Could you check a few things on this model? Use its own coordinates, in mm. Face numbers are marked on the shaded views. Coordinates: 2 decimals unless noted, no trailing zeros. Loops run counter-clockwise (first coordinate to the right, second up) from the corner with the lowest first, then second, coordinate; pieces in that order, holes last. Notation, with made-up numbers: (51.25, 42) - (68.25, 42) arc R17 ccw to (68.25, 69) - close; hole circle Ø3 at (-7, -19.5). An arc over 180 degrees is marked (long way). Put each result on its own line as item: value. Start each with the question number.
Autodesk Inventor part; units mm, degrees
ref_plane "YZ Plane" through (0, 0, 0) normal (1, 0, 0) x (0, 1, 0)
ref_plane "XZ Plane" through (0, 0, 0) normal (0, 1, 0) x (-1, 0, 0)
ref_plane "XY Plane" through (0, 0, 0) normal (0, 0, 1) x (1, 0, 0)
sketch "Sketch1" plane through (0, 0, 0) normal (0, 1, 0) x (-1, 0, 0)
  line L0 (113.8016, -163.8079) -> (118.6285, -172.1682)
  line L1 (113.8016, -163.8079) -> (118.4883, -163.8079)
  arc A0 (32.1771, -413.0024) -> (33.3318, -411.0024) centre (32.1771, -411.669) ccw
  line L2 (26.4886, -397.8099) -> (26.4886, -373.629)
  arc A1 (26.4886, -370.9624) -> (26.4886, -373.629) centre (26.4886, -372.2957) ccw
  line L3 (26.4886, -370.9624) -> (32.9886, -370.9624)
  arc A2 (32.9886, -373.629) -> (32.9886, -370.9624) centre (32.9886, -372.2957) ccw
  line L4 (32.9886, -373.629) -> (32.9886, -380.9624)
  line L5 (-88.7072, -380.9624) -> (-33.5061, -380.9624)
  line L6 (32.9886, -380.9624) -> (90.3221, -380.9624)
  arc A3 (-33.9776, -411.0024) -> (-32.8229, -413.0024) centre (-32.8229, -411.669) ccw
  arc A4 (-27.1344, -373.6228) -> (-27.0061, -370.9624) centre (-27.0061, -372.2957) ccw
  line L7 (-27.0061, -370.9624) -> (-33.5061, -370.9624)
  arc A5 (-33.5061, -370.9624) -> (-33.5061, -373.629) centre (-33.5061, -372.2957) ccw
  line L8 (-33.5061, -373.629) -> (-33.5061, -380.9624)
  line L9 (118.4883, -148.1364) -> (118.4883, -161.1412)
  line L10 (33.3318, -411.0024) -> (27.1585, -400.3099)
  arc A6 (26.4886, -397.8099) -> (27.1585, -400.3099) centre (31.4886, -397.8099) ccw
  line L11 (-27.1344, -397.8099) -> (-27.1344, -373.6228)
  line L12 (-33.9776, -411.0024) -> (-27.8043, -400.3099)
  arc A7 (-27.8043, -400.3099) -> (-27.1344, -397.8099) centre (-32.1344, -397.8099) ccw
  line L13 (-32.8229, -413.0024) -> (32.1771, -413.0024)
  line L14 (-11.4601, -148.0629) -> (-11.4601, -168.7264)
  line L15 (156.6836, -142.6364) -> (162.6836, -142.6364)
  line L16 (162.6836, -142.6364) -> (162.6836, -148.1364)
  line L17 (156.6866, -148.1364) -> (118.4883, -148.1364)
  line L18 (11.6836, -145.4697) -> (11.6846, -142.6364)
  line L19 (11.6846, -142.6364) -> (5.6846, -142.6364)
  line L20 (5.6846, -142.6364) -> (5.6845, -148.1281)
  line L21 (11.6831, -148.1364) -> (49.8814, -148.1364)
  arc A8 (11.6836, -145.4697) -> (11.6831, -148.1364) centre (11.6831, -146.803) ccw
  arc A9 (3.0194, -148.0629) -> (5.6845, -148.1281) centre (4.3512, -148.1281) ccw
  line L22 (-11.4601, -148.0629) -> (3.0194, -148.0629)
  line L23 (-11.4601, -171.393) -> (-18.9601, -171.393)
  arc A10 (-11.4601, -171.393) -> (-11.4601, -168.7264) centre (-11.4601, -170.0597) ccw
  line L24 (162.6836, -145.3864) -> (185.043, -145.3864) construction
  line L25 (21.6753, -413.0028) -> (-28.7481, -413.0028) construction
  line L26 (-0.3229, -413.0028) -> (-0.3229, -413.0028)
  arc A11 (-89.9069, -379.0472) -> (-88.7072, -380.9624) centre (-88.7072, -379.629) ccw
  line L27 (156.6836, -142.6364) -> (156.6836, -145.4697)
  line L28 (165.3503, -148.1364) -> (179.8299, -148.1364)
  arc A12 (156.6866, -148.1364) -> (156.6836, -145.4697) centre (156.6836, -146.803) ccw
  arc A13 (162.6836, -148.1364) -> (165.3503, -148.1364) centre (164.017, -148.1364) ccw
  line L29 (179.8299, -148.1364) -> (179.8299, -171.4697)
  line L30 (179.8299, -171.4697) -> (172.3299, -171.4697)
  line L31 (90.3221, -380.9624) -> (90.3221, -378.9624)
  line L32 (90.3221, -376.2957) -> (97.8221, -376.2957)
  arc A14 (90.3221, -376.2957) -> (90.3221, -378.9624) centre (90.3221, -377.629) ccw
  line L33 (118.4883, -161.1412) -> (118.4883, -164.2811)
  arc A15 (118.4883, -163.8079) -> (118.4883, -161.1412) centre (118.4883, -162.4745) ccw
  line L34 (84.1849, -148.1364) -> (84.1849, -155.2534)
  arc A16 (117.4738, -174.1682) -> (118.6285, -172.1682) centre (117.4738, -172.8349) ccw
  line L35 (84.1849, -174.1682) -> (117.4738, -174.1682)
  line L36 (54.5681, -163.8079) -> (49.7413, -172.1682)
  line L37 (54.5681, -163.8079) -> (49.8814, -163.8079)
  line L38 (49.8814, -148.1364) -> (49.8814, -161.1412)
  line L39 (49.8814, -161.1412) -> (49.8814, -164.2811)
  arc A17 (49.8814, -161.1412) -> (49.8814, -163.8079) centre (49.8814, -162.4745) ccw
  arc A18 (49.7413, -172.1682) -> (50.896, -174.1682) centre (50.896, -172.8349) ccw
  line L40 (84.1849, -174.1682) -> (50.896, -174.1682)
  arc A19 (97.8221, -376.2957) -> (172.3299, -171.4697) centre (-250.9666, -133.4553) ccw
  arc A20 (-89.9069, -379.0472) -> (-18.9601, -171.393) centre (-669.0585, -65.2283) ccw
  point P0 (-90.8396, -380.9624)
  point P1 (-27.3048, -399.1039)
  dimension "d102" = 2.6667
  dimension "d107" = 2.6667
  dimension "d108" = 6.5
  dimension "d109" = 2.6667
  dimension "d141" = 7.3333
  dimension "d142" = 5
  dimension "d170" = 13.0048
  dimension "d173" = 6
  dimension "d174" = 5.5
  dimension "d177" = 7.5
  dimension "d179" = 2.6667
  dimension "d181" = 232.826
  dimension "d183" = 264.8664
  dimension "d184" = 23.3301
  dimension "d186" = 57.3335
  dimension "d187" = 57.3335
  dimension "d189" = 6.5
  dimension "d190" = 7.3333
  dimension "d191" = 24.187
  dimension "d192" = 1.3333
  dimension "d202" = 6
  dimension "d203" = 1.3333
  dimension "d204" = 1.3333
  dimension "d208" = 191.29
  dimension "d209" = 2.6667
  dimension "d210" = 2.6667
  dimension "d211" = 14.4796
  dimension "d212" = 14.4796
  dimension "d213" = 61.3416
  dimension "d214" = 145
  dimension "d216" = 23.3333
  dimension "d217" = 7.5
  dimension "d220" = 7.5
  dimension "d221" = 2.6667
  dimension "d223" = 38.1984
  dimension "d226" = 61.3416
  dimension "d232" = 2.6667
  dimension "d233" = 2.6667
  dimension "d234" = 61.3416
  dimension "d235" = 60
  dimension "d236" = 33.2889
  dimension "d237" = 2
  dimension "d238" = 425
  dimension "d239" = 658.71
extrude "Extrusion4" add sketch "Sketch1" along normal blind 6 contours L1 A15 L9 L17 A12 L27 L15 L16 A13 L28 L29 L30 A19 L32 A14 L31 L6 L4 A2 L3 A1 L2 A6 L10 A0 L13 A3 L12 A7 L11 A4 L7 A5 L8 L5 A11 A20 L23 A10 L14 L22 A9 L20 L19 L18 A8 L21 L38 A17 L37 L36 A18 L40 L35 A16 L0
properties part number "Support C"
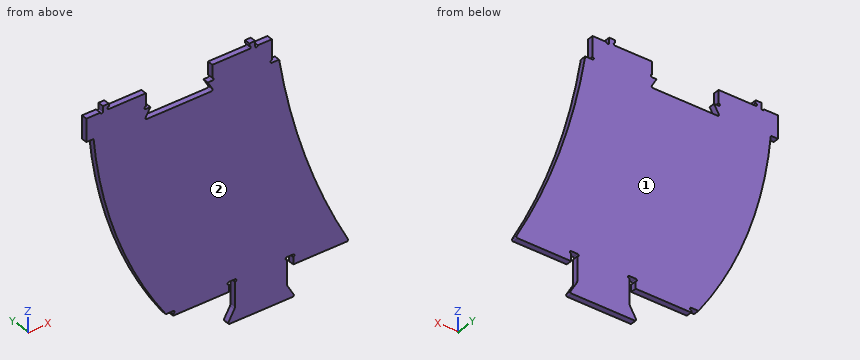
(1) For pin 1 Ø3 at (y, z) = (1, -281.5) entering from -X; pin 2 Ø2.5 at (y, z) = (4, -144) entering from -X; pin 3 Ø1.8 at (x, y) = (-77.5, 2) entering from +Z, each with a flat end and sliding along its axis, tell me the tip position at first contact or that it passes through.
(2) I want a section at B-B on z = -339. List the corners of the cut face in (x, y) for me.
(3) I need wall thicknesses on L1, parallel to X at y = 3.7, z = -372; L2, parallel to X at y = 4.4, z = -156.5; L3, parallel to X at y = 4.95, z = -375. Which ranges of each line are inside material? Lowest first, please. Write a range as [from, to].
(4) I want a section at A-A on x = -80.5. List the corners of the cut face in (y, z) for me, and give its area (3 significant figures).
(5) If we mould it in two halves opening along Y, with no side actions, what happens to the marked faces 1 and 2? For each: pulls with the +Y half, pulls with the -Y half, needs draft (parallel to the pull), parting line crosses it, or undercut.
Answer sheet:
1. pin 1: stops at x = -147.97
1. pin 2: stops at x = -162.68
1. pin 3: stops at z = -174.17
2. outline: (-121.02, 0) - (69.94, 0) - (69.94, 6) - (-121.02, 6) - close
3. L1: x = [-100.77, -34.29], [-25.19, 25.71], [34.81, 86.14]
3. L2: x = [-179.83, -118.49], [-49.88, 11.46]
3. L3: x = [-98.72, -32.99], [-26.49, 27.13], [33.51, 87.73]
4. outline: (0, -380.96) - (6, -380.96) - (6, -174.17) - (0, -174.17) - close
4. area: 1,240 mm^2
5. face 1: pulls with the +Y half
5. face 2: pulls with the -Y half
